Geometry check sheet. Reference: the model listing, model coordinates, mm. Round coordinates to 2 decimals unless told otherwise and drop trailing zeros. Write each loop counter-clockwise with the first axis right and the second up, starting at its lowest first coordinate (ties: lowest second). Pieces come first, ordered by that corner, then holes. Notation, with made-up numbers: (35, -1) -> (68, -1) arc R26 ccw to (68, 33) -> close; hole circle Ø2 at (86, -36). An arc over 180 degrees is marked (long way). Put each result on its own line as item: value. Start each with the question number.
from build123d import *

# Parameters (mm, degrees)
SKETCH1_W           = 3
SKETCH1_H           = 10
BOSS_EXTRUDE1_DEPTH = 3


with BuildPart() as part:
    # Sketch1 → Boss-Extrude1 (new body)
    with BuildSketch(Plane.XY):
        Polygon((-74.5, 61.9), (-55, 61.9), (-55, 64.9), (-45, 64.9), (-45, 61.9), (-5, 61.9), (-5, 64.9), (5, 64.9), (5, 61.9), (45, 61.9), (45, 64.9), (55, 64.9), (55, 61.9), (74.5, 61.9), (74.5, 12.5), (84.5, 12.5), (84.5, -12.5), (74.5, -12.5), (74.5, -67.1), (65, -67.1), (65, -70.1), (55, -70.1), (55, -67.1), (35, -67.1), (35, -70.1), (25, -70.1), (25, -67.1), (5, -67.1), (5, -70.1), (-5, -70.1), (-5, -67.1), (-25, -67.1), (-25, -70.1), (-35, -70.1), (-35, -67.1), (-55, -67.1), (-55, -70.1), (-65, -70.1), (-65, -67.1), (-74.5, -67.1), (-74.5, -12.5), (-84.5, -12.5), (-84.5, 12.5), (-74.5, 12.5), align=None)
        with Locations((73, 0)):
            Rectangle(SKETCH1_W, SKETCH1_H, mode=Mode.SUBTRACT)
        with Locations((-73, 0)):
            Rectangle(SKETCH1_W, SKETCH1_H, mode=Mode.SUBTRACT)
    extrude(amount=BOSS_EXTRUDE1_DEPTH)


solid = part.part
(1) Sectioned sample at B-B (z = 1.6). State how many separate pieces and enclosed holes the cut face has, and give its area (3 significant figures).
(2) Sectioned sample at A-A (y = -3). Record the cut outline in (x, z), and give its area (3 significant figures).
(3) Go/stop test with flat-tipped pins: pin 1 Ø1 at (y, z) = (-48.5, 1) entering from +X; pin 2 Ø0.9 at (y, z) = (-68, 1) entering from -X; pin 3 Ø1.5 at (x, y) = (0.5, -49) entering from -Z; pin 4 Ø1.5 at (x, z) = (-79, 2) entering from -Y. Record where each tip stops, or that it passes through.
(4) Material ranges on L1, parallel to X at y = 3, z = 0.4; L2, parallel to X at y = -37, z = 0.3; L3, parallel to Y at x = -27.5, z = 1.7, recorded low to high. Write a range as from..to.
(5) Sectioned sample at C-C (x = -31). Record the cut outline in (y, z).
(6) Sectioned sample at D-D (y = 33). Record the cut outline in (x, z).
Found:
1. separate pieces: 1
1. enclosed holes: 2
1. area: 19,900 mm2
2. outline: (-84.5, 0) -> (-74.5, 0) -> (-74.5, 3) -> (-84.5, 3) -> close; (-71.5, 0) -> (71.5, 0) -> (71.5, 3) -> (-71.5, 3) -> close; (74.5, 0) -> (84.5, 0) -> (84.5, 3) -> (74.5, 3) -> close
2. area: 489 mm2
3. pin 1: x = 74.5
3. pin 2: x = -65
3. pin 3: z = 0
3. pin 4: y = -12.5
4. L1: -84.5..-74.5, -71.5..71.5, 74.5..84.5
4. L2: -74.5..74.5
4. L3: -70.1..61.9
5. outline: (-70.1, 0) -> (61.9, 0) -> (61.9, 3) -> (-70.1, 3) -> close
6. outline: (-74.5, 0) -> (74.5, 0) -> (74.5, 3) -> (-74.5, 3) -> close
